Input: part model. Units: mm. Frame: model coordinates. A direction names the side the tool comes from. Coordinates: 2 decimals unless noted, no trailing zeros.
from build123d import *

# Parameters (mm, degrees)
SKETCH_1_R          = 1.6
EXTRUDE_1_DEPTH     = 5
CUT_EXTRUDE_1_DEPTH = 10
SKETCH_3_R          = 1.85
CUT_EXTRUDE_2_DEPTH = 10
SKETCH_4_R          = 10.25
CUT_EXTRUDE_3_DEPTH = 10
SKETCH_5_RX         = 62.536642564
SKETCH_5_RY         = 23.496138081
CUT_EXTRUDE_4_DEPTH = 10
FILLET_1_R          = 10
CUT_EXTRUDE_5_DEPTH = 10
CUT_EXTRUDE_6_DEPTH = 10
CUT_EXTRUDE_7_DEPTH = 10
CUT_EXTRUDE_8_DEPTH = 10
CUT_EXTRUDE_9_DEPTH = 10


with BuildPart() as part:
    # 草图1 → 凸台-拉伸1 (new body)
    with BuildSketch(Plane.XY):
        with BuildLine():
            Line((100, -150), (-100, -150))
            Line((-100, -150), (-100, 100))
            ThreePointArc((-100, 100), (-85.355339059, 135.355339059), (-50, 150))
            Line((-50, 150), (50, 150))
            ThreePointArc((50, 150), (85.355339059, 135.355339059), (100, 100))
            Line((100, 100), (100, -150))
        make_face()
        with Locations((-34.521960573, -8.188147907)):
            Circle(SKETCH_1_R, mode=Mode.SUBTRACT)
        with Locations((17.550731265, -3.107088494)):
            Circle(SKETCH_1_R, mode=Mode.SUBTRACT)
        with Locations((16.284685109, -51.357276396)):
            Circle(SKETCH_1_R, mode=Mode.SUBTRACT)
        with Locations((-34.521960573, -36.128147907)):
            Circle(SKETCH_1_R, mode=Mode.SUBTRACT)
    extrude(amount=-EXTRUDE_1_DEPTH)

    # 草图2 → 切除-拉伸1 (cut)
    with BuildSketch(Plane.XY):
        with BuildLine():
            Line((-77.5, 93.5), (-77.5, 95))
            Line((-77.5, 95), (-76, 95))
            ThreePointArc((-76, 95), (-78.560660172, 96.060660172), (-77.5, 93.5))
        make_face()
        with BuildLine():
            Line((-76, 95), (-77.5, 95))
            Line((-77.5, 95), (-77.5, 93.5))
            ThreePointArc((-77.5, 93.5), (-76.439339828, 93.939339828), (-76, 95))
        make_face()
        with BuildLine():
            ThreePointArc((-76, 65), (-76.439339828, 66.060660172), (-77.5, 66.5))
            Line((-77.5, 66.5), (-77.5, 65))
            Line((-77.5, 65), (-76, 65))
        make_face()
        with BuildLine():
            Line((-77.5, 65), (-77.5, 66.5))
            ThreePointArc((-77.5, 66.5), (-78.560660172, 63.939339828), (-76, 65))
            Line((-76, 65), (-77.5, 65))
        make_face()
        with BuildLine():
            ThreePointArc((84, 95), (82.5, 96.5), (81, 95))
            Line((81, 95), (82.5, 95))
            Line((82.5, 95), (82.5, 93.5))
            ThreePointArc((82.5, 93.5), (83.560660172, 93.939339828), (84, 95))
        make_face()
        with BuildLine():
            Line((82.5, 95), (81, 95))
            ThreePointArc((81, 95), (81.439339828, 93.939339828), (82.5, 93.5))
            Line((82.5, 93.5), (82.5, 95))
        make_face()
        with BuildLine():
            ThreePointArc((84, 65), (83.560660172, 66.060660172), (82.5, 66.5))
            Line((82.5, 66.5), (82.5, 65))
            Line((82.5, 65), (81, 65))
            ThreePointArc((81, 65), (82.5, 63.5), (84, 65))
        make_face()
        with BuildLine():
            Line((82.5, 65), (82.5, 66.5))
            ThreePointArc((82.5, 66.5), (81.439339828, 66.060660172), (81, 65))
            Line((81, 65), (82.5, 65))
        make_face()
        with BuildLine():
            ThreePointArc((84, -80), (82.5, -78.5), (81, -80))
            Line((81, -80), (82.5, -80))
            Line((82.5, -80), (82.5, -81.5))
            ThreePointArc((82.5, -81.5), (83.560660172, -81.060660172), (84, -80))
        make_face()
        with BuildLine():
            Line((82.5, -80), (81, -80))
            ThreePointArc((81, -80), (81.439339828, -81.060660172), (82.5, -81.5))
            Line((82.5, -81.5), (82.5, -80))
        make_face()
        with BuildLine():
            ThreePointArc((84, -110), (83.560660172, -108.939339828), (82.5, -108.5))
            Line((82.5, -108.5), (82.5, -110))
            Line((82.5, -110), (81, -110))
            ThreePointArc((81, -110), (82.5, -111.5), (84, -110))
        make_face()
        with BuildLine():
            Line((82.5, -110), (82.5, -108.5))
            ThreePointArc((82.5, -108.5), (81.439339828, -108.939339828), (81, -110))
            Line((81, -110), (82.5, -110))
        make_face()
        with BuildLine():
            ThreePointArc((-76, -110), (-76.439339828, -108.939339828), (-77.5, -108.5))
            Line((-77.5, -108.5), (-77.5, -110))
            Line((-77.5, -110), (-76, -110))
        make_face()
        with BuildLine():
            Line((-77.5, -110), (-77.5, -108.5))
            ThreePointArc((-77.5, -108.5), (-78.560660172, -111.060660172), (-76, -110))
            Line((-76, -110), (-77.5, -110))
        make_face()
        with BuildLine():
            Line((-77.5, -81.5), (-77.5, -80))
            Line((-77.5, -80), (-76, -80))
            ThreePointArc((-76, -80), (-78.560660172, -78.939339828), (-77.5, -81.5))
        make_face()
        with BuildLine():
            Line((-76, -80), (-77.5, -80))
            Line((-77.5, -80), (-77.5, -81.5))
            ThreePointArc((-77.5, -81.5), (-76.439339828, -81.060660172), (-76, -80))
        make_face()
    extrude(amount=-CUT_EXTRUDE_1_DEPTH, mode=Mode.SUBTRACT)

    # 草图3 → 切除-拉伸2 (cut)
    with BuildSketch(Plane.XY):
        with Locations((-5, 105)):
            Circle(SKETCH_3_R)
        with Locations((5, 105)):
            Circle(SKETCH_3_R)
        with Locations((-5, 57)):
            Circle(SKETCH_3_R)
        with Locations((5, 57)):
            Circle(SKETCH_3_R)
    extrude(amount=-CUT_EXTRUDE_2_DEPTH, mode=Mode.SUBTRACT)

    # 草图4 → 切除-拉伸3 (cut)
    with BuildSketch(Plane.XY):
        with Locations((-68.667685953, -128.956279274)):
            Circle(SKETCH_4_R)
    extrude(amount=-CUT_EXTRUDE_3_DEPTH, mode=Mode.SUBTRACT)

    # 草图5 → 切除-拉伸4 (cut)
    with BuildSketch(Plane.XY):
        with Locations((0, -150)):
            Ellipse(SKETCH_5_RX, SKETCH_5_RY)
    extrude(amount=-CUT_EXTRUDE_4_DEPTH, mode=Mode.SUBTRACT)

    # 圆角1
    fillet_1_edges = [part.edges().sort_by_distance(p)[0] for p in [
        (100, -150, -2.5),
        (62.536642564, -150, -2.5),
        (-62.536642564, -150, -2.5),
        (-100, -150, -2.5),
    ]]
    fillet(fillet_1_edges, radius=FILLET_1_R)

    # 草图6 → 切除-拉伸5 (cut)
    with BuildSketch(Plane.XY):
        Polygon((44.756616737, 68.037030505), (37.194996558, 81.134140843), (44.756616737, 94.231251181), (59.879857096, 94.231251181), (67.441477275, 81.134140843), (59.879857096, 68.037030505), align=None)
        Polygon((-37.194996558, 81.134140843), (-44.756616737, 94.231251181), (-59.879857096, 94.231251181), (-67.441477275, 81.134140843), (-59.879857096, 68.037030505), (-44.756616737, 68.037030505), align=None)
    extrude(amount=-CUT_EXTRUDE_5_DEPTH, mode=Mode.SUBTRACT)

    # 草图9 → 切除-拉伸6 (cut)
    with BuildSketch(Plane.XY):
        Polygon((-83, 35), (-100, 41.187493983), (-100, 14.740188926), align=None)
        Polygon((-83, 8.552694943), (-100, 14.740188926), (-100, -11.707116131), align=None)
        Polygon((-83, -17.894610113), (-100, -11.707116131), (-100, -38.154421187), align=None)
        Polygon((-81.191926789, -45), (-100, -38.154421187), (-100, -67.414588819), align=None)
        Polygon((100, -38.154421187), (81.191926789, -45), (100, -67.414588819), align=None)
        Polygon((83, -17.894610113), (100, -38.154421187), (100, -11.707116131), align=None)
        Polygon((83, 8.552694943), (100, -11.707116131), (100, 14.740188926), align=None)
        Polygon((83, 35), (100, 14.740188926), (100, 41.187493983), align=None)
    extrude(amount=-CUT_EXTRUDE_6_DEPTH, mode=Mode.SUBTRACT)

    # 草图10 → 切除-拉伸7 (cut)
    with BuildSketch(Plane.XY):
        Polygon((10, 27), (5, 35.660254038), (-5, 35.660254038), (-10, 27), (-5, 18.339745962), (5, 18.339745962), align=None)
        Polygon((10, -66.503861919), (5, -57.843607881), (-5, -57.843607881), (-10, -66.503861919), (-5, -75.164115957), (5, -75.164115957), align=None)
    extrude(amount=-CUT_EXTRUDE_7_DEPTH, mode=Mode.SUBTRACT)

    # 草图12 → 切除-拉伸8 (cut)
    with BuildSketch(Plane(origin=(0, 0, -5), x_dir=(-1, 0, 0), z_dir=(0, 0, -1))):
        with BuildLine():
            ThreePointArc((-85.355339059, 135.355339059), (-96.193976626, 119.134171618), (-100, 100))
            Line((-100, 100), (-85.355339059, 135.355339059))
        make_face()
        with BuildLine():
            ThreePointArc((-50, 150), (-69.134171618, 146.193976626), (-85.355339059, 135.355339059))
            Line((-85.355339059, 135.355339059), (-50, 150))
        make_face()
        with BuildLine():
            ThreePointArc((85.355339059, 135.355339059), (69.134171618, 146.193976626), (50, 150))
            Line((50, 150), (85.355339059, 135.355339059))
        make_face()
        with BuildLine():
            Line((85.355339059, 135.355339059), (100, 100))
            ThreePointArc((100, 100), (96.193976626, 119.134171618), (85.355339059, 135.355339059))
        make_face()
    extrude(amount=-CUT_EXTRUDE_8_DEPTH, mode=Mode.SUBTRACT)

    # 草图13 → 切除-拉伸9 (cut)
    with BuildSketch(Plane(origin=(0, 0, -5), x_dir=(-1, 0, 0), z_dir=(0, 0, -1))):
        with BuildLine():
            Line((-41.29, 131.8), (-34.29, 131.8))
            ThreePointArc((-34.29, 131.8), (-32.69, 133.4), (-34.29, 135))
            Line((-34.29, 135), (-41.29, 135))
            ThreePointArc((-41.29, 135), (-42.89, 133.4), (-41.29, 131.8))
        make_face()
        with BuildLine():
            ThreePointArc((34.29, 131.8), (32.69, 133.4), (34.29, 135))
            Line((34.29, 135), (41.29, 135))
            ThreePointArc((41.29, 135), (42.89, 133.4), (41.29, 131.8))
            Line((41.29, 131.8), (34.29, 131.8))
        make_face()
    extrude(amount=-CUT_EXTRUDE_9_DEPTH, mode=Mode.SUBTRACT)


solid = part.part
Item 1: Draft query along X for faces 1 (the face through (-92.575, 117.925, -2.535)), 2 (the face through (-41.03, 74.49, -2.46)), 3 (the face through (1, 2, -5)). Return one class per face: pulls with the +X half, pulls with the -X half, needs draft (parallel to the pull), parting line crosses it, or undercut.
Response values:
face 1: pulls with the -X half
face 2: undercut
face 3: needs draft
Item 2: Cut plane A-A on z = -2.8. Count the separate pieces of the cut face and the enclosed holes in it, then the cut area to 3 significant figures.
Response values:
separate pieces: 1
enclosed holes: 23
area: 52,000 mm2
Item 3: Ray query, probe 1 along Y at (x, z) = (-60, -4.65); probe 2 along X at (y, z) = (95, -2.7); probe 3 along Y at (x, z) = (-91, -0.85). Return the intervals inside material, ascending.
Response values:
probe 1: y = -143.38 to -134.43, -123.49 to 68.25, 94.02 to 145.86
probe 2: x = -100 to -79, -76 to 81, 84 to 100
probe 3: y = -149.95 to -56.69, -41.43 to -27.43, -14.98 to -0.98, 11.46 to 25.47, 37.91 to 121.73
Item 4: Access query for faces 4 (the face through (96.99, -147.15, -2.54)), 5 (the face through (91.38, -27.88, -2.46)), 6 (the face through (63.61, 87.77, -2.46)), 7 (the face through (-91.62, -28.17, -2.46)). Directions: +Z, -Z, +X, -X, +Y, -Y. A direction counts if a zero-diameter tool reaches every point of the face in a straight line with its end or side. Return the directions, or none.
Response values:
face 4: +Z, -Z, +X, -Y
face 5: +Z, -Z, +X
face 6: +Z, -Z
face 7: +Z, -Z, -X
Item 5: Pin query (flat end, axial travel): pin 1 Ø18.5 at (x, y) = (-68.67, -128.96) entering from +Z; pin 2 Ø3.5 at (x, y) = (-77.5, -110) entering from -Z; pin 3 Ø1.5 at (x, z) = (-36.5, -2.5) entering from -Y. Return the tip coordinate at first contact, or that it passes through.
Response values:
pin 1: passes through
pin 2: stops at z = -5
pin 3: stops at y = -131.13
